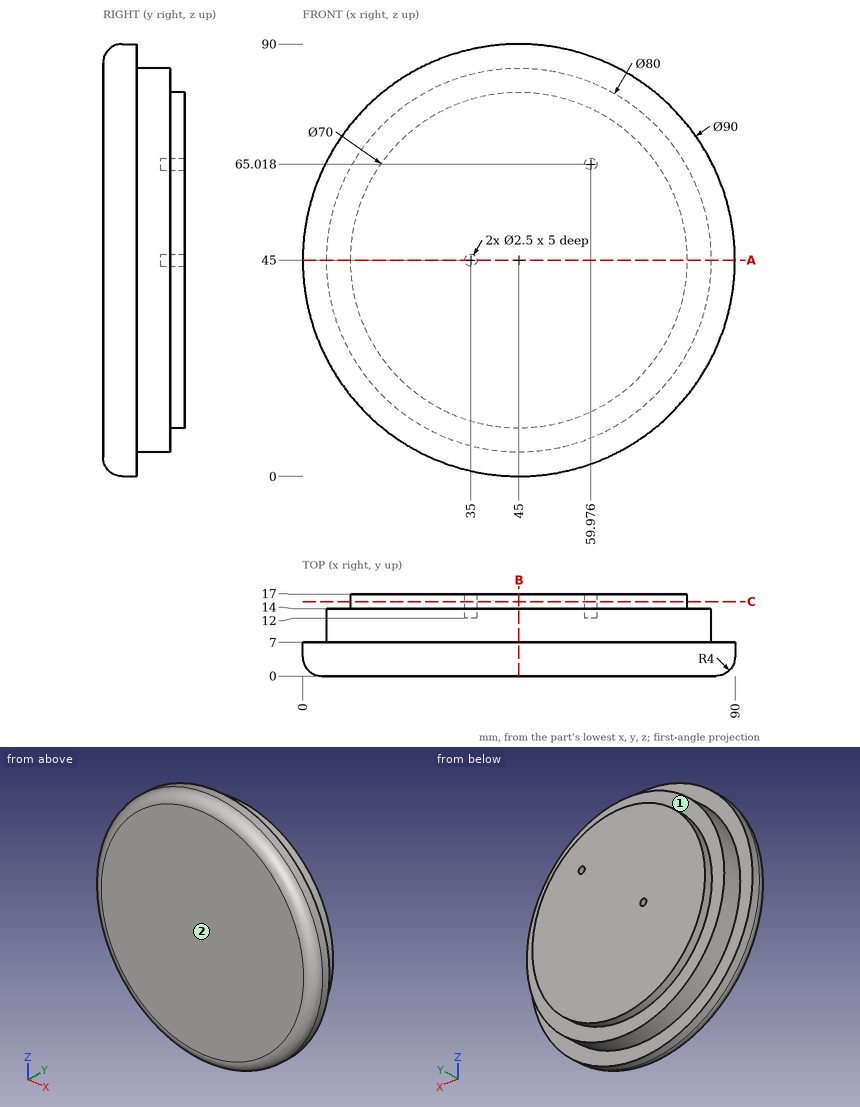
Study the drawing (mm; zero at the part's minimum x, y, z) and answer. A direction names the side the tool comes from. Round coordinates to 2 decimals unless told otherwise and drop trailing zeros. Order: outer loops, then holes, each group sorted by start corner. A loop starts at its lowest first (then second) coordinate and runs counter-clockwise, first axis right, second up. Notation, with made-up numbers: (87, 15.25) - (136, 15.25) arc R29 ccw to (136, 35.25) - close; hole circle Ø3 at (67, 82.25). An arc over 180 degrees is marked (long way). Use one line per item in the form item = value. Start each with the question number.
(1) The part is cut by section B-B (x = 45). Give the vertices of the cut face in (y, z), then the cut area to 3 significant figures.
(2) The part is cut by section A-A (z = 45). Give the vertices of the cut face in (x, y).
(3) Find the intervals of material crossed by line 1 along Y through (x, z) = (25, 76); line 2 along Z through (x, y) = (35, 13.1); line 3 along Z through (x, y) = (71, 2.5), in increasing order. Write a range as from..to.
(4) Flat-ended cylindrical pins translate along their axes: pin 1 Ø1.5 at (x, y) = (58, 13.5) entering from +Z; pin 2 Ø0.8 at (x, z) = (35, 45.5) entering from +Y; pin 3 Ø8 at (y, z) = (8.5, 28.5) entering from +X. Find the tip coordinate at first contact, or state that the pin passes through.
(5) The part is cut by section C-C (y = 15.5). Give the vertices of the cut face in (x, z), then the cut area to 3 significant figures.
(6) For the marked faces 1 and 2, determine the directions among +Z, -Z, +X, -X, +Y, -Y from which every point of the face is accessible in a straight line to the end or side of a thin tool.
Checked values:
q1.outline = (0, 4) arc R4 ccw to (4, 0) - (7, 0) - (7, 5) - (14, 5) - (14, 10) - (17, 10) - (17, 80) - (14, 80) - (14, 85) - (7, 85) - (7, 90) - (4, 90) arc R4 ccw to (0, 86) - close
q1.area = 1,390 mm^2
q2.outline = (0, 4) arc R4 ccw to (4, 0) - (86, 0) arc R4 ccw to (90, 4) - (90, 7) - (85, 7) - (85, 14) - (80, 14) - (80, 17) - (36.25, 17) - (36.25, 12) - (33.75, 12) - (33.75, 17) - (10, 17) - (10, 14) - (5, 14) - (5, 7) - (0, 7) - close
q3.line_1 = 0..14
q3.line_2 = 6.27..43.75, 46.25..83.73
q3.line_3 = 8.63..81.37
q4.pin_1 = 83.08
q4.pin_2 = 12
q4.pin_3 = 88.14
q5.outline = circle Ø70 at (45, 45); hole circle Ø2.5 at (35, 45); hole circle Ø2.5 at (59.98, 65.02)
q5.area = 3,840 mm^2
q6.face_1 = +Y
q6.face_2 = +Z, -Z, +X, -X, -Y
